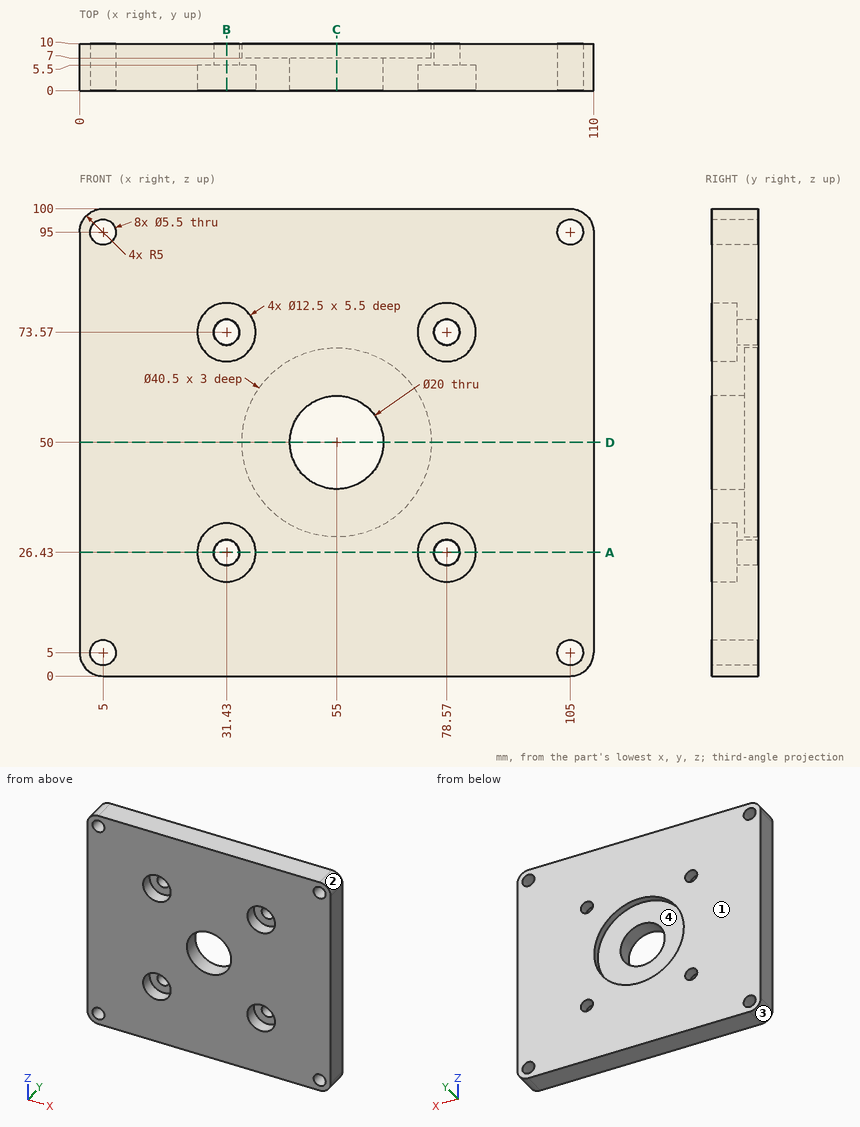
Answer from the drawing. Dimensions are ordinates in mm from the lowest x, y and z of the part. Round coordinates to 2 decimals unless told otherwise and drop trailing zeros. Write each loop counter-clockwise with the first axis right and the second up, starting at its lowest first coordinate (ties: lowest second). Pieces come first, ordered by that corner, then holes. Notation, with made-up numbers: M 75,-6.75 L 128,-6.75 A35 ccw 128,26.25 Z; hole C 76.25,-6.5 d8. An arc over 180 degrees is marked long. Write each question's results on one line, items separated by ' | '. Start each with the question number.
Item 1: Flat-ended cylindrical pins translate along their axes: pin 1 Ø7 at (x, z) = (31.43, 26.43) entering from -Y; pin 2 Ø12 at (x, z) = (62, 41) entering from +Y. Find the tip coordinate at first contact, or state that the pin passes through.
Item 2: A cutting plane is placed at C-C on x = 55. Write down the section's boundary in (y, z).
Item 3: A cutting plane is placed at D-D on z = 50. Write down the section's boundary in (x, y).
Item 4: A cutting plane is placed at A-A on z = 26.43. Write down the section's boundary in (x, y), and give its area (3 significant figures).
Item 5: For a pull along X with two mould halves and no side action, classify the marked faces 1, 2, 3 and 4 as pulls with the +X half, pulls with the -X half, needs draft (parallel to the pull), parting line crosses it, or undercut.
Item 6: Straight lines are drawn through the part: L1, parallel to X at y = 7.5, z = 26.43; L2, parallel to Z at x = 31.43, y = 7.95; L3, parallel to X at y = 1.75, z = 26.43. For each, find the intervals that lie inside material, in ascending order. Write a range as [from, to].
Item 7: A cutting plane is placed at B-B on x = 31.43. Write down the section's boundary in (y, z), and give its area (3 significant figures).
Check sheet entries:
1) pin 1: y = 5.5 | pin 2: y = 7
2) outline: M 0,0 L 10,0 L 10,29.75 L 7,29.75 L 7,40 L 0,40 Z; M 0,60 L 7,60 L 7,70.25 L 10,70.25 L 10,100 L 0,100 Z
3) outline: M 0,0 L 45,0 L 45,7 L 34.75,7 L 34.75,10 L 0,10 Z; M 65,0 L 110,0 L 110,10 L 75.25,10 L 75.25,7 L 65,7 Z
4) outline: M 0,0 L 25.18,0 L 25.18,5.5 L 28.68,5.5 L 28.68,10 L 0,10 Z; M 34.18,5.5 L 37.68,5.5 L 37.68,0 L 72.32,0 L 72.32,5.5 L 75.82,5.5 L 75.82,10 L 34.18,10 Z; M 81.32,5.5 L 84.82,5.5 L 84.82,0 L 110,0 L 110,10 L 81.32,10 Z | area: 913 mm²
5) face 1: needs draft | face 2: pulls with the +X half | face 3: pulls with the -X half | face 4: undercut
6) L1: [0, 28.68], [34.18, 75.82], [81.32, 110] | L2: [0, 23.68], [29.18, 70.82], [76.32, 100] | L3: [0, 25.18], [37.68, 72.32], [84.82, 110]
7) outline: M 0,0 L 10,0 L 10,23.68 L 5.5,23.68 L 5.5,20.18 L 0,20.18 Z; M 0,32.68 L 5.5,32.68 L 5.5,29.18 L 10,29.18 L 10,70.82 L 5.5,70.82 L 5.5,67.32 L 0,67.32 Z; M 0,79.82 L 5.5,79.82 L 5.5,76.32 L 10,76.32 L 10,100 L 0,100 Z | area: 813 mm²
